Geometry check sheet. Reference: drawing and pictorial views, mm from the part's lowest x, y, z. A direction names the side the tool comes from. Coordinates: 2 decimals unless noted, no trailing zeros. Loops run counter-clockwise (first coordinate to the right, second up) from the corner with the lowest first, then second, coordinate; pieces in that order, holes last.
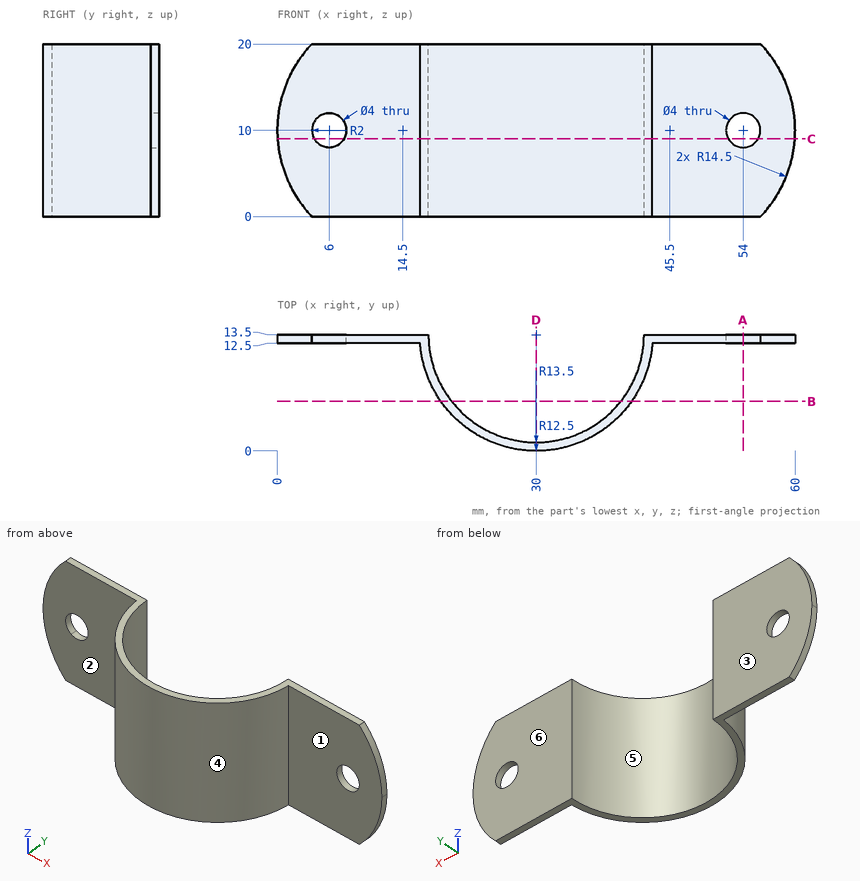
1) Mould release check, pull along X, two halves, no side actions. Record for the marked faces 4, 5 and 6: +X half, -X half, draft (parallel to the pull), parting line (faces both ways), or undercut.
Data:
face 4: parting line
face 5: undercut
face 6: draft
2) Section check B-B on y = 5.75. Record the cut outline in (x, z).
Data:
outline: (18.95, 0) - (20.19, 0) - (20.19, 20) - (18.95, 20) - close; (39.81, 0) - (41.05, 0) - (41.05, 20) - (39.81, 20) - close
3) Section check A-A on x = 54. Record the cut outline in (y, z).
Data:
outline: (12.5, 0) - (13.5, 0) - (13.5, 8) - (12.5, 8) - close; (12.5, 12) - (13.5, 12) - (13.5, 20) - (12.5, 20) - close
4) Depth check by flat-ended pin: pin 1 (8.5 mm diameter, centred on x = 8, z = 13.5, fed in from -Y); pin 2 (1 mm diameter, centred on y = 10.5, z = 17, fed in from -X); pin 3 (3 mm diameter, centred on x = 6, z = 10, fed in from +Y); pin 4 (8 mm diameter, centred on y = 7, z = 3.5, fed in from +X). Enter the tip coordinate at first touch or a pass-through.
Data:
pin 1: stops at y = 12.5
pin 2: stops at x = 16.73
pin 3: passes through
pin 4: stops at x = 43.27
5) Section check D-D on x = 30. Record the cut outline in (y, z), and give its area (3 significant figures).
Data:
outline: (0, 0) - (1, 0) - (1, 20) - (0, 20) - close
area: 20.0 mm2
6) Material ranges on probe 1 along Z at (x, y) = (6, 12.85); probe 2 along Y at (x, z) = (4, 15.75); probe 3 along X at (y, z) = (8.25, 6.75), recorded low to high.
Data:
probe 1: z = 0 to 8, 12 to 20
probe 2: y = 12.5 to 13.5
probe 3: x = 17.56 to 18.66, 41.34 to 42.44
7) Access from +Z, -Z, +X, -X, +Y, -Y to the whole of each face (thin tool, end or side, straight path). Record for the marked faces 1, 2 and 3.
Data:
face 1: +Z, -Z, +X, -Y
face 2: +Z, -Z, -X, -Y
face 3: +Z, -Z, +X, -X, +Y
8) Section check C-C on z = 9. Record the cut outline in (x, y), and give its area (3 significant figures).
Data:
outline: (0.03, 12.5) - (4.27, 12.5) - (4.27, 13.5) - (0.03, 13.5) - close; (7.73, 12.5) - (16.54, 12.5) arc R13.5 ccw to (43.46, 12.5) - (52.27, 12.5) - (52.27, 13.5) - (42.5, 13.5) arc R12.5 cw to (17.5, 13.5) - (7.73, 13.5) - close; (55.73, 12.5) - (59.97, 12.5) - (59.97, 13.5) - (55.73, 13.5) - close
area: 66.9 mm2
